from build123d import *

# Parameters (mm, degrees)
SKETCH1_R           = 304.8
BOSS_EXTRUDE1_DEPTH = 88.9
SKETCH2_R           = 16.51
CUT_EXTRUDE6_DEPTH  = 88.9


with BuildPart() as part:
    # Sketch1 → Boss-Extrude1 (new body)
    with BuildSketch(Plane.XY):
        Circle(SKETCH1_R)
    extrude(amount=BOSS_EXTRUDE1_DEPTH)

    # Sketch2 → Cut-Extrude6 (cut)
    with BuildSketch(Plane.XY.offset(88.9)):
        with Locations((0, 266.7)):
            Circle(SKETCH2_R)
        with Locations((69.027039329, 257.612417871)):
            Circle(SKETCH2_R)
        with Locations((133.35, 230.968975189)):
            Circle(SKETCH2_R)
        with Locations((188.585378542, 188.585378542)):
            Circle(SKETCH2_R)
        with Locations((230.968975189, 133.35)):
            Circle(SKETCH2_R)
        with Locations((257.612417871, 69.027039329)):
            Circle(SKETCH2_R)
        with Locations((266.7, 0)):
            Circle(SKETCH2_R)
        with Locations((257.612417871, -69.027039329)):
            Circle(SKETCH2_R)
        with Locations((230.968975189, -133.35)):
            Circle(SKETCH2_R)
        with Locations((188.585378542, -188.585378542)):
            Circle(SKETCH2_R)
        with Locations((133.35, -230.968975189)):
            Circle(SKETCH2_R)
        with Locations((69.027039329, -257.612417871)):
            Circle(SKETCH2_R)
        with Locations((0, -266.7)):
            Circle(SKETCH2_R)
        with Locations((-69.027039329, -257.612417871)):
            Circle(SKETCH2_R)
        with Locations((-133.35, -230.968975189)):
            Circle(SKETCH2_R)
        with Locations((-188.585378542, -188.585378542)):
            Circle(SKETCH2_R)
        with Locations((-230.968975189, -133.35)):
            Circle(SKETCH2_R)
        with Locations((-257.612417871, -69.027039329)):
            Circle(SKETCH2_R)
        with Locations((-266.7, 0)):
            Circle(SKETCH2_R)
        with Locations((-257.612417871, 69.027039329)):
            Circle(SKETCH2_R)
        with Locations((-230.968975189, 133.35)):
            Circle(SKETCH2_R)
        with Locations((-188.585378542, 188.585378542)):
            Circle(SKETCH2_R)
        with Locations((-133.35, 230.968975189)):
            Circle(SKETCH2_R)
        with Locations((-69.027039329, 257.612417871)):
            Circle(SKETCH2_R)
    extrude(amount=-CUT_EXTRUDE6_DEPTH, mode=Mode.SUBTRACT)


solid = part.part
For this review, take the finished solid that the model builds, in its own axes (mm). Coordinates: 2 decimals unless noted, no trailing zeros. Order: outer loops, then holes, each group sorted by start corner. A loop starts at its lowest first (then second) coordinate and runs counter-clockwise, first axis right, second up. Notation, with made-up numbers: (64, -11) - (111, -11) arc R22 cw to (111, 15) - close; hole circle Ø3 at (46, -16). An arc over 180 degrees is marked (long way). Use one line per item in the form item = value.
Q1. Draft analysis for pull direction X (two halves, no side actions). For faces 1 (the cylindrical face through (141, -245.6, 45.1)), 2 (the flat face through (-4, 4, 0)), 3 (the cylindrical face through (-241.879, -185.466, 43.828)), state which applies: +X half, -X half, draft (parallel to the pull), parting line (faces both ways), or undercut.
Checked values:
face_1 = undercut
face_2 = draft
face_3 = parting line
Q2. For P1, Ø10, axis at x = 163.5, y = 8.5, coming from the -Z side; P2, Ø8, axis at y = -113.5, z = 72.5, coming from the -X side; P3, Ø1, axis at x = -201, z = 33, coming from the +Y side; P4, Ø2, axis at y = 108, z = 18, coming from the +X side, all flat-tipped, find the tip position at first contact; note any pin that passes through.
Checked values:
P1 = 0
P2 = -284.45
P3 = 229.57
P4 = 285.4
Q3. Consider section B-B (x = -266.7). Give the boundary of the cut face in (y, z).
Checked values:
outline = (-147.56, 0) - (-82.81, 0) - (-82.81, 88.9) - (-147.56, 88.9) - close; (-55.24, 0) - (-16.51, 0) - (-16.51, 88.9) - (-55.24, 88.9) - close; (16.51, 0) - (55.24, 0) - (55.24, 88.9) - (16.51, 88.9) - close; (82.81, 0) - (147.56, 0) - (147.56, 88.9) - (82.81, 88.9) - close
Q4. Consider section A-A (x = 0). Give the boundary of the cut face in (y, z), then the cut area to 3 significant figures.
Checked values:
outline = (-304.8, 0) - (-283.21, 0) - (-283.21, 88.9) - (-304.8, 88.9) - close; (-250.19, 0) - (250.19, 0) - (250.19, 88.9) - (-250.19, 88.9) - close; (283.21, 0) - (304.8, 0) - (304.8, 88.9) - (283.21, 88.9) - close
area = 48,300 mm2
Q5. Consider section C-C (z = 21). Give the number of separate pieces and of enclosed holes in the cut face, then the cut area to 3 significant figures.
Checked values:
separate_pieces = 1
enclosed_holes = 24
area = 271,000 mm2
Q6. For probe 1 along X at (y, z) = (-133, 31); probe 2 along X at (y, z) = (-74, 53); probe 3 along Y at (x, z) = (143.5, 12), list the stretches that pass through material, from the lowest coordinate up. Write a range as from..to.
Checked values:
probe_1 = -274.25..-247.48, -214.46..214.46, 247.48..274.25
probe_2 = -295.68..-273.36, -241.87..241.87, 273.36..295.68
probe_3 = -268.91..-243.99, -217.95..217.95, 243.99..268.91
